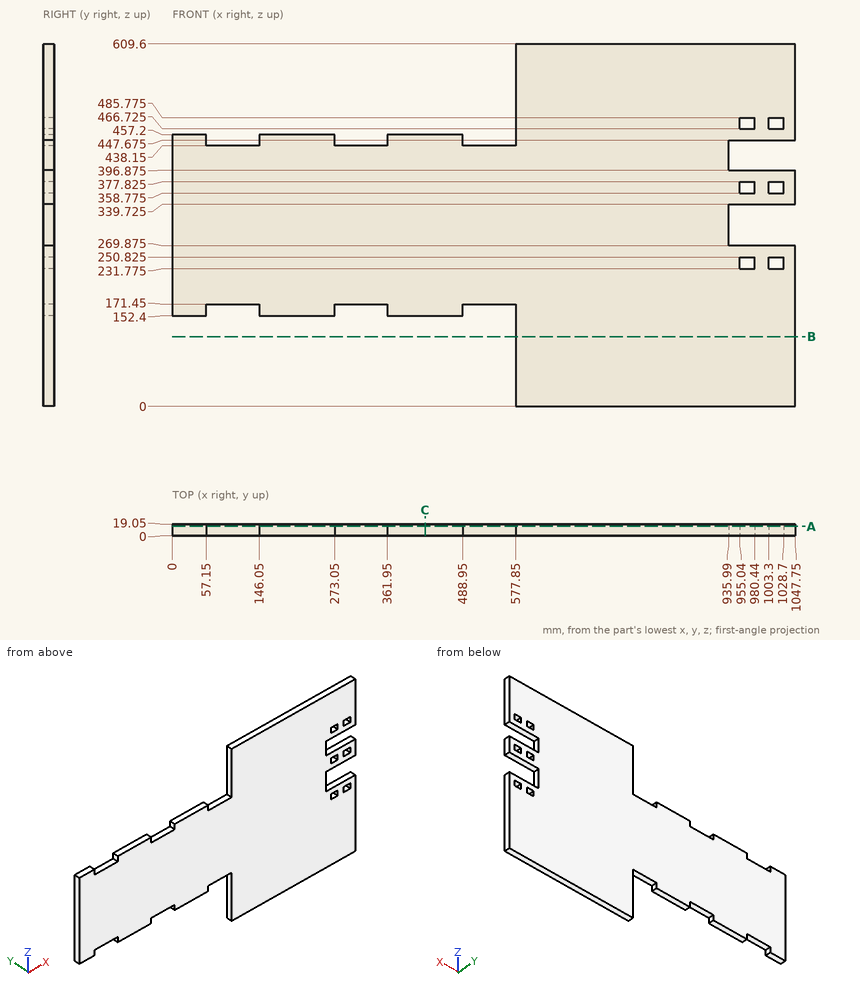
Print and shaded views of the part. All mm, measured from the part's lowest x, y and z. Give positions to 0.01 mm unless a question says otherwise; leave off trailing zeros. Write each loop counter-clockwise with the first axis right and the second up, starting at its lowest first coordinate (ties: lowest second). Pieces come first, ordered by that corner, then holes. Notation, with made-up numbers: M -6.5,16.25 L 34.5,16.25 A26 cw 34.5,54.25 Z; hole C 36.25,-36.75 d1. An arc over 180 degrees is marked long. Use a Markdown table: item, result.
1) Cut at B-B (z = 117). List the corners of the cut face in (x, y), and give its area (3 significant figures).
Responses:
| item | result |
|---|---|
| outline | M 577.85,0 L 1047.75,0 L 1047.75,19.05 L 577.85,19.05 Z |
| area | 8,950 mm2 |
2) Cut at A-A (y = 15.5). Give the number of separate pieces and of enclosed holes in the cut face, and give its area (3 significant figures).
Responses:
| item | result |
|---|---|
| separate pieces | 1 |
| enclosed holes | 6 |
| area | 436,000 mm2 |
3) Cut at C-C (x = 425.5). List the corners of the cut face in (y, z).
Responses:
| item | result |
|---|---|
| outline | M 0,152.4 L 19.05,152.4 L 19.05,457.2 L 0,457.2 Z |
4) Pin check, flat tips, straight feed: pin 1 (5.5 mm diameter, centred on x = 227.5, y = 13.5, fed in from -Z); pin 2 (10 mm diameter, centred on x = 272.5, y = 15.5, fed in from +Z); pin 3 (9.5 mm diameter, centred on y = 9, z = 302, fed in from +X). Stop position of each tip, or through.
Responses:
| item | result |
|---|---|
| pin 1 | stops at z = 152.4 |
| pin 2 | stops at z = 457.2 |
| pin 3 | stops at x = 935.99 |
5) Drill centre lines: line 1 (X direction, y = 8, z = 238); line 2 (Z direction, x = 535, y = 1); line 3 (X direction, y = 3.5, z = 285). Where is each one in solid material? Low to high. Write a range as from..to.
Responses:
| item | result |
|---|---|
| line 1 | x = 0..955.04, 980.44..1003.3, 1028.7..1047.75 |
| line 2 | z = 171.45..438.15 |
| line 3 | x = 0..935.99 |
